from build123d import *

# Parameters (mm, degrees)
CUT_EXTRUDE1_DEPTH  = 8.5
BOSS_EXTRUDE1_DEPTH = 3
FILLET1_R           = 3


with BuildPart() as part:
    # Sketch1 → Revolve1 (revolve)
    with BuildSketch(Plane(origin=(0, 0, 0), x_dir=(0, 0, -1), z_dir=(1, 0, 0))):
        Polygon((-2, 0), (-13, 0), (-13, -1), (-14, -1), (-14, -11), (-12, -11), (-12, -2), (-2, -2), align=None)
    revolve(axis=Axis((0, 0, 0), (0, -1, 0)))

    # Sketch3 → Cut-Extrude1 (cut)
    with BuildSketch(Plane.XY.offset(13)):
        with BuildLine():
            Line((1, -9), (-1, -9))
            ThreePointArc((-1, -9), (-3.17855614, -8.354682272), (-4.654181831, -6.626946572))
            Line((-4.654181831, -6.626946572), (-7.159459855, -1))
            Line((-7.159459855, -1), (7.159459855, -1))
            Line((7.159459855, -1), (4.654181831, -6.626946572))
            ThreePointArc((4.654181831, -6.626946572), (3.17855614, -8.354682272), (1, -9))
        make_face()
    extrude(amount=CUT_EXTRUDE1_DEPTH, mode=Mode.SUBTRACT)

    # Sketch4 → Boss-Extrude1 (add, symmetric)
    with BuildSketch(Plane(origin=(0, 0, 0), x_dir=(0, 0, -1), z_dir=(1, 0, 0))):
        with BuildLine():
            Line((13, -1), (16, -1))
            ThreePointArc((16, -1), (18.331437884, 0.112038827), (18.934442802, 2.623735072))
            Line((18.934442802, 2.623735072), (18.31070773, 5.558177875))
            Line((18.31070773, 5.558177875), (19.28885533, 5.766089565))
            Line((19.28885533, 5.766089565), (19.912590403, 2.831646763))
            ThreePointArc((19.912590403, 2.831646763), (19.108583846, -0.517281564), (16, -2))
            Line((16, -2), (13, -2))
            Line((13, -2), (13, -1))
        make_face()
    extrude(amount=BOSS_EXTRUDE1_DEPTH, both=True)

    # Sketch5 → Revolve2 (revolve)
    with BuildSketch(Plane(origin=(0, 0, 0), x_dir=(0, 0, -1), z_dir=(1, 0, 0)), mode=Mode.PRIVATE) as revolve2_sk:
        Polygon((18.518619421, 4.580030274), (27.321947827, 6.451235491), (24.411184156, 20.145301902), (22.454888954, 19.72947852), (24.949829244, 7.991707311), (19.08094364, 6.744237166), (19.28885533, 5.766089565), (18.31070773, 5.558177875), align=None)
    revolve(revolve2_sk.sketch.rotate(Axis((0, 20.145301902, -24.411184156), (0, -0.20791169081776387, 0.9781476007338047)), 180), axis=Axis((0, 20.145301902, -24.411184156), (0, -0.20791169081776387, 0.9781476007338047)))

    # Fillet1
    fillet1_edges = [part.edges().sort_by_distance(p)[0] for p in [
        (0, 6.451235491, -27.321947827),
        (0, 7.991707311, -24.949829244),
    ]]
    fillet(fillet1_edges, radius=FILLET1_R)

    # Sketch6 → Revolve3 (revolve)
    with BuildSketch(Plane(origin=(0, 0, 0), x_dir=(0, 0, -1), z_dir=(1, 0, 0))):
        with BuildLine():
            Line((0.75, 1), (0.75, -0.75))
            ThreePointArc((0.75, -0.75), (1.116116524, -1.633883476), (2, -2))
            Line((2, -2), (2, 0))
            ThreePointArc((2, 0), (1.469669914, 0.219669914), (1.25, 0.75))
            Line((1.25, 0.75), (1.25, 1))
            Line((1.25, 1), (0.75, 1))
        make_face()
    revolve(axis=Axis((0, 0, 0), (0, 1, 0)))

    # Sketch7 → Revolve4 (revolve)
    with BuildSketch(Plane(origin=(0, 0, 0), x_dir=(0, 0, -1), z_dir=(1, 0, 0)), mode=Mode.PRIVATE) as revolve4_sk:
        with BuildLine():
            Line((22.454888954, 19.72947852), (17.560305242, 18.689102635))
            Line((17.560305242, 18.689102635), (17.404371474, 19.422713336))
            Line((17.404371474, 19.422713336), (19.853586184, 19.943309993))
            ThreePointArc((19.853586184, 19.943309993), (21.430483377, 21.027081408), (21.779175959, 22.908458222))
            Line((21.779175959, 22.908458222), (22.454888954, 19.72947852))
        make_face()
    revolve(revolve4_sk.sketch.rotate(Axis((0, 19.72947852, -22.454888954), (0, -0.20791169081776406, 0.9781476007338047)), 192.373625116), axis=Axis((0, 19.72947852, -22.454888954), (0, -0.20791169081776406, 0.9781476007338047)))


solid = part.part
Could you check a few things on this model? Use its own coordinates, in mm. A direction names the side the tool comes from. Give positions to 0.01 mm unless a question says otherwise; leave off trailing zeros. Order: outer loops, then holes, each group sorted by start corner. A loop starts at its lowest first (then second) coordinate and runs counter-clockwise, first axis right, second up.
1. Thinking about a two-plate mould opening in X: for faces 4 (the cylindrical face through (8.52, -6.07, -11.11)), 5 (the flat face through (8.606, 10.064, -18.375)), 6 (the cylindrical face through (0.04, -0.48, -19.14)), which applies, +X half, -X half, draft (parallel to the pull), parting line (faces both ways), or undercut?
Answers below:
face 4: parting line
face 5: undercut
face 6: draft
2. Which directions (+Z, -Z, +X, -X, +Y, -Y) give clear straight access to the entire face, cutting with the end or side of a thin tool? Please do faces 1 (the flat face through (-0.1, -1, -13.2)), 2 (the cylindrical face through (0.042, 0.083, -18.308)), 3 (the cylindrical face through (-0.53, -6.44, -11.99)).
Answers below:
face 1: none
face 2: +X, -X
face 3: -Y
3. Suppose I cut it at A-A (z = 0). Write out the boundary of the cut face in (x, y), plus the area to 3 significant figures.
Answers below:
outline: (-14, -11) - (-12, -11) - (-12, -2) - (-2, -2) arc R1.25 ccw to (-0.75, -0.75) - (-0.75, 1) - (-1.25, 1) - (-1.25, 0.75) arc R0.75 cw to (-2, 0) - (-13, 0) - (-13, -1) - (-14, -1) - close; (0.75, -0.75) arc R1.25 ccw to (2, -2) - (12, -2) - (12, -11) - (14, -11) - (14, -1) - (13, -1) - (13, 0) - (2, 0) arc R0.75 cw to (1.25, 0.75) - (1.25, 1) - (0.75, 1) - close
area: 87.6 mm2
4. For pin 1 (12 mm diameter, centred on x = -4, y = 0.5, fed in from -Z); pin 2 (0.8 mm diameter, centred on x = 0, z = 0.5, fed in from +Y); pin 3 (1.9 mm diameter, centred on y = 2, z = -17.5, fed in from +X); pin 4 (6 mm diameter, centred on x = -3, z = 0.5, fed in from -Y), each with a flat end and sliding along its axis, tell me the tip position at first contact or that it passes through.
Answers below:
pin 1: stops at z = -25.09
pin 2: stops at y = 1
pin 3: passes through
pin 4: stops at y = -2
5. I need wall thicknesses on L1, parallel to X at y = -4, z = 0; L2, parallel to X at y = -0.25, z = 0; L3, parallel to Z at x = 0, y = -0.3. Which ranges of each line are inside material? Lowest first, please.
Answers below:
L1: x = -14 to -12, 12 to 14
L2: x = -13 to -0.75, 0.75 to 13
L3: z = -19.27 to -17.93, -13 to -0.75, 0.75 to 13
6. Suppose I cut it at C-C (z = 8). Write out the boundary of the cut face in (x, y).
Answers below:
outline: (-11.49, -11) - (-8.94, -11) - (-8.94, -2) - (8.94, -2) - (8.94, -11) - (11.49, -11) - (11.49, -1) - (10.25, -1) - (10.25, 0) - (-10.25, 0) - (-10.25, -1) - (-11.49, -1) - close
7. Suppose I cut it at B-B (z = -5.5). Write out the boundary of the cut face in (x, y).
Answers below:
outline: (-12.87, -11) - (-10.67, -11) - (-10.67, -2) - (10.67, -2) - (10.67, -11) - (12.87, -11) - (12.87, -1) - (11.78, -1) - (11.78, 0) - (-11.78, 0) - (-11.78, -1) - (-12.87, -1) - close
